Geometry check sheet. Reference: the model listing, model coordinates, mm. Round coordinates to 2 decimals unless told otherwise and drop trailing zeros. Order: outer loops, then holes, each group sorted by start corner. A loop starts at its lowest first (then second) coordinate and runs counter-clockwise, first axis right, second up. Notation, with made-up numbers: (61.25, -39) - (112.25, -39) arc R32 ccw to (112.25, 0) - close; hole circle Ø10 at (20.25, -8). An arc over 180 degrees is marked (long way). Return JSON: item names as keys, results as strings. Group by question number.
Q1. Sectioned sample at C-C, the plane y = -12.5. Record the cut outline in (x, z).
Q2. Gauge pin test, flat ends, axial feed: pin 1 Ø2 at (x, z) = (-1, 2.5) entering from +Y; pin 2 Ø2 at (y, z) = (15.5, 2.5) entering from +X; pin 3 Ø1.2 at (y, z) = (-22, 2) entering from -X. Record the tip position at first contact, or that the pin passes through.
Q3. Sectioned sample at A-A, the plane z = 2.2. Record the cut outline in (x, y), then the cut area to 3 significant figures.
Q4. Sectioned sample at B-B, the plane x = 31. Record the cut outline in (y, z).
Q5. Material ranges on line 1 along Y through (x, z) = (-35, 2.9); line 2 along X through (y, z) = (16, 2.8), recorded low to high.
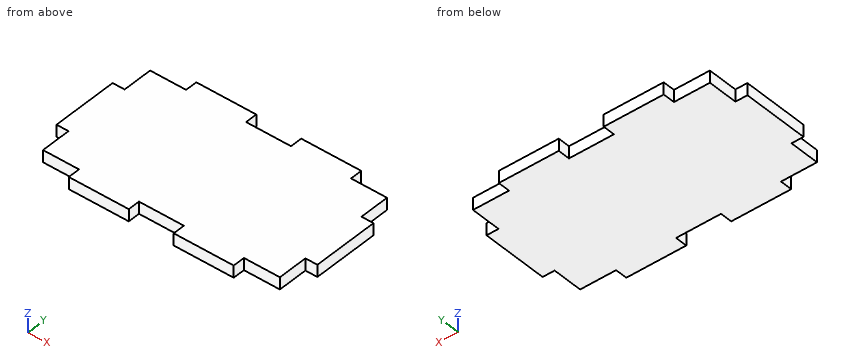
Autodesk Inventor part; units mm, degrees
ref_plane "YZ Plane" through (0, 0, 0) normal (1, 0, 0) x (0, 1, 0)
ref_plane "XZ Plane" through (0, 0, 0) normal (0, 1, 0) x (-1, 0, 0)
ref_plane "XY Plane" through (0, 0, 0) normal (0, 0, 1) x (1, 0, 0)
sketch "Эскиз1" plane through (0, 0, 0) normal (0, 0, 1) x (1, 0, 0)
  line L0 (0, -21) -> (-7.5, -21)
  line L1 (-7.5, -21) -> (-7.5, -25)
  line L2 (-7.5, -25) -> (-27.5, -25)
  line L3 (-27.5, -25) -> (-27.5, -21)
  line L4 (-27.5, -21) -> (-39.5, -21)
  line L5 (-39.5, -21) -> (-39.5, -11)
  line L6 (-39.5, -11) -> (-43.5, -11)
  line L7 (-43.5, -11) -> (-43.5, 0)
  line L8 (-43.5, 0) -> (0, 0)
  line L9 (0, 21) -> (-7.5, 21)
  line L10 (-7.5, 21) -> (-7.5, 25)
  line L11 (-7.5, 25) -> (-27.5, 25)
  line L12 (-27.5, 25) -> (-27.5, 21)
  line L13 (-27.5, 21) -> (-39.5, 21)
  line L14 (-39.5, 21) -> (-39.5, 11)
  line L15 (-39.5, 11) -> (-43.5, 11)
  line L16 (-43.5, 11) -> (-43.5, 0)
  line L17 (0, -21) -> (0, 21)
  line L18 (0, -21) -> (7.5, -21)
  line L19 (7.5, -21) -> (7.5, -25)
  line L20 (7.5, -25) -> (27.5, -25)
  line L21 (27.5, -25) -> (27.5, -21)
  line L22 (27.5, -21) -> (39.5, -21)
  line L23 (39.5, -21) -> (39.5, -11)
  line L24 (39.5, -11) -> (43.5, -11)
  line L25 (43.5, -11) -> (43.5, 0)
  line L26 (43.5, 0) -> (0, 0)
  line L27 (0, 21) -> (7.5, 21)
  line L28 (7.5, 21) -> (7.5, 25)
  line L29 (7.5, 25) -> (27.5, 25)
  line L30 (27.5, 25) -> (27.5, 21)
  line L31 (27.5, 21) -> (39.5, 21)
  line L32 (39.5, 21) -> (39.5, 11)
  line L33 (39.5, 11) -> (43.5, 11)
  line L34 (43.5, 11) -> (43.5, 0)
  dimension "d1" = 20
  dimension "d3" = 12
  dimension "d4" = 22
  dimension "d5" = 4
  dimension "d6" = 10
  dimension "d7" = 15
extrude "Выдавливание1" add sketch "Эскиз1" along normal blind 4
properties part number "batMain" material "Дерево (береза)"
Reply:
{
 "1": {"outline": "(-39.5, 0) - (39.5, 0) - (39.5, 4) - (-39.5, 4) - close"},
 "2": {"pin 1": "y = 21", "pin 2": "x = 39.5", "pin 3": "x = -27.5"},
 "3": {"outline": "(-43.5, -11) - (-39.5, -11) - (-39.5, -21) - (-27.5, -21) - (-27.5, -25) - (-7.5, -25) - (-7.5, -21) - (7.5, -21) - (7.5, -25) - (27.5, -25) - (27.5, -21) - (39.5, -21) - (39.5, -11) - (43.5, -11) - (43.5, 11) - (39.5, 11) - (39.5, 21) - (27.5, 21) - (27.5, 25) - (7.5, 25) - (7.5, 21) - (-7.5, 21) - (-7.5, 25) - (-27.5, 25) - (-27.5, 21) - (-39.5, 21) - (-39.5, 11) - (-43.5, 11) - close", "area": "3,810 mm^2"},
 "4": {"outline": "(-21, 0) - (21, 0) - (21, 4) - (-21, 4) - close"},
 "5": {"line 1": "-21 to 21", "line 2": "-39.5 to 39.5"}
}
